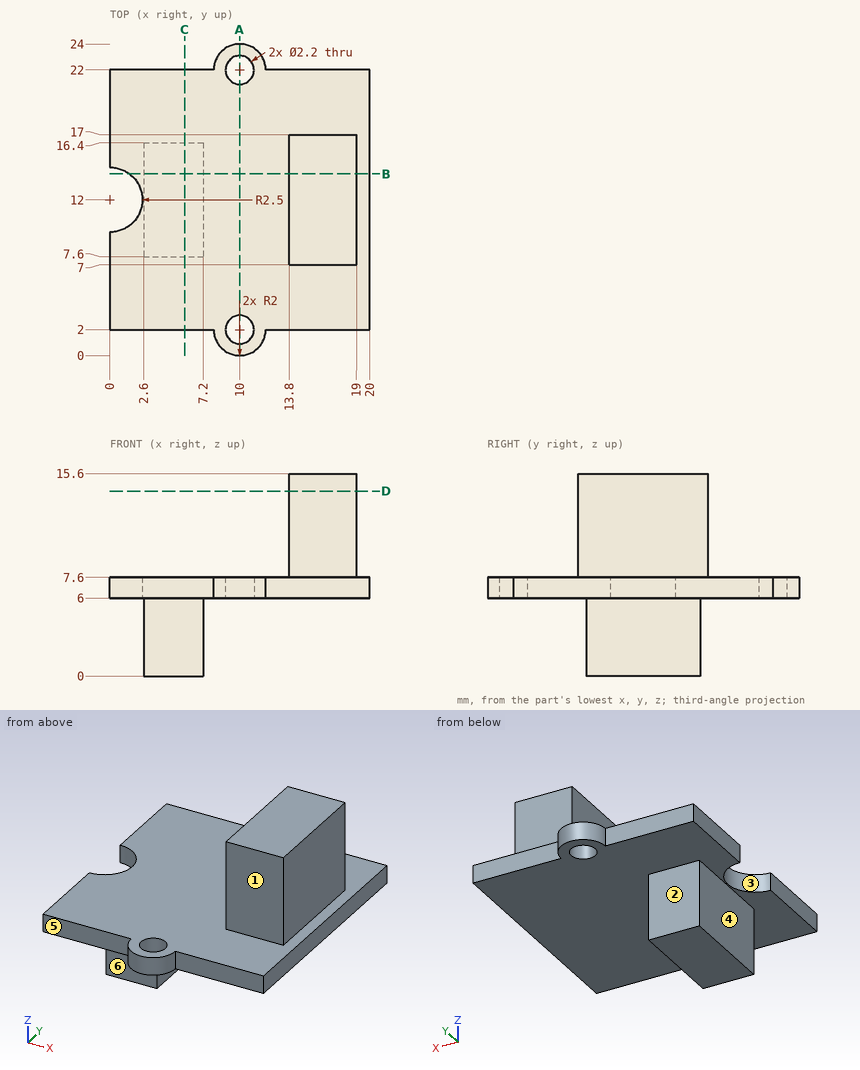
The drawing under review shows one solid part. Ordinate dimensions are in mm from its lowest x, y, z. A direction names the side the tool comes from. Round coordinates to 2 decimals unless told otherwise and drop trailing zeros. Loops run counter-clockwise (first coordinate to the right, second up) from the corner with the lowest first, then second, coordinate; pieces in that order, holes last. Notation, with made-up numbers: (45.25, 7) -> (58.25, 7) arc R17 ccw to (58.25, 24) -> close; hole circle Ø5 at (36, 85). An arc over 180 degrees is marked (long way). Answer in a Markdown table with one row per item.
1) Consider section C-C, the plane x = 5.75. Write out the cut boundary in (y, z).
Taken from the geometry:
| item | result |
|---|---|
| outline | (2, 6) -> (7.6, 6) -> (7.6, 0) -> (16.4, 0) -> (16.4, 6) -> (22, 6) -> (22, 7.6) -> (2, 7.6) -> close |
2) Wall thickness on line 1 along Y through (x, z) = (10, 6.65); line 2 along X through (y, z) = (10.25, 1.5); line 3 along Y through (x, z) = (15.25, 11.5): over which ranges is each line inside the solid? List them lowest first.
Taken from the geometry:
| item | result |
|---|---|
| line 1 | y = 0 to 0.9, 3.1 to 20.9, 23.1 to 24 |
| line 2 | x = 2.6 to 7.2 |
| line 3 | y = 7 to 17 |
3) For pin 1 Ø4 at (x, z) = (15, 10.5) entering from -Y; pin 2 Ø0.5 at (x, z) = (4, 7) entering from +Y; pin 3 Ø9 at (y, z) = (14, 13) entering from -X, all flat-tipped, find the tip position at first contact; note any pin that passes through.
Taken from the geometry:
| item | result |
|---|---|
| pin 1 | stops at y = 7 |
| pin 2 | stops at y = 22 |
| pin 3 | stops at x = 13.8 |
4) Consider section B-B, the plane y = 14. Write out the cut boundary in (x, z).
Taken from the geometry:
| item | result |
|---|---|
| outline | (1.5, 6) -> (2.6, 6) -> (2.6, 0) -> (7.2, 0) -> (7.2, 6) -> (20, 6) -> (20, 7.6) -> (19, 7.6) -> (19, 15.6) -> (13.8, 15.6) -> (13.8, 7.6) -> (1.5, 7.6) -> close |
5) Draft analysis for pull direction Y (two halves, no side actions). For the marked faces 1, 2 and 3, state which applies: pulls with the +Y half, pulls with the -Y half, needs draft (parallel to the pull), parting line crosses it, or undercut.
Taken from the geometry:
| item | result |
|---|---|
| face 1 | pulls with the -Y half |
| face 2 | pulls with the +Y half |
| face 3 | undercut |
6) Consider section D-D, the plane z = 14.25. Write out the cut boundary in (x, y).
Taken from the geometry:
| item | result |
|---|---|
| outline | (13.8, 7) -> (19, 7) -> (19, 17) -> (13.8, 17) -> close |
7) Consider section A-A, the plane x = 10. Write out the cut boundary in (y, z), plus the area to 3 significant figures.
Taken from the geometry:
| item | result |
|---|---|
| outline | (0, 6) -> (0.9, 6) -> (0.9, 7.6) -> (0, 7.6) -> close; (3.1, 6) -> (20.9, 6) -> (20.9, 7.6) -> (3.1, 7.6) -> close; (23.1, 6) -> (24, 6) -> (24, 7.6) -> (23.1, 7.6) -> close |
| area | 31.4 mm² |
8) Tool access review of the marked faces 4, 5 and 6: name each direction out of +Z, -Z, +X, -X, +Y, -Y from which nothing blocks a thin tool from reaching the whole face with its end or side.
Taken from the geometry:
| item | result |
|---|---|
| face 4 | -Z, -X, +Y, -Y |
| face 5 | +Z, -Z, -X, -Y |
| face 6 | -Z, +X, -X, -Y |
